Check sheet for the modelled part. Datum: model origin and axes. Units: mm. Face numbers are marked on the shaded views. A direction names the side the tool comes from. Round coordinates to 2 decimals unless told otherwise and drop trailing zeros. Loops run counter-clockwise (first coordinate to the right, second up) from the corner with the lowest first, then second, coordinate; pieces in that order, holes last. Notation, with made-up numbers: (26, 77) -> (38, 77) arc R15 ccw to (38, 102) -> close; hole circle Ø7 at (22, 58). An arc over 180 degrees is marked (long way). Return JSON: item names as keys, results as strings.
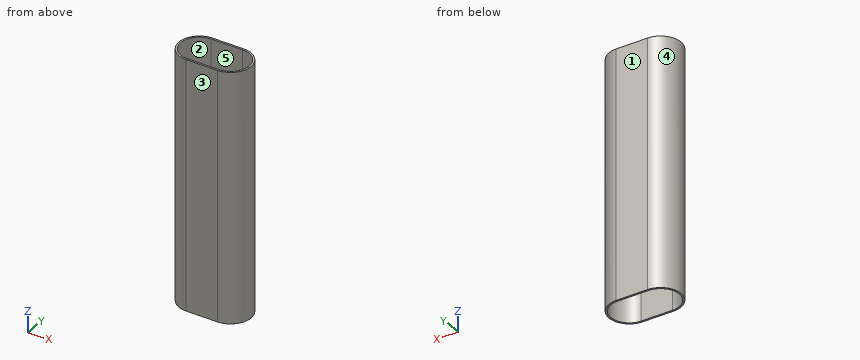
from build123d import *

# Parameters (mm, degrees)
F1_DEPTH = 85
F0_W     = 50
F0_H     = 7
F2_R     = 12.5
F2_R_2   = 7.5
F3_DEPTH = 12.5
F4_W     = 25.6223708915
F4_H     = 20
F5_DEPTH = 25


with BuildPart() as f1:
    # F0 (on Top) → F1 (new body)
    with BuildSketch(Plane.XY):
        with BuildLine():
            Line((5.35, 6.9), (-5.35, 6.9))
            ThreePointArc((-5.35, 6.9), (-12.25, 0), (-5.35, -6.9))
            Line((-5.35, -6.9), (5.35, -6.9))
            ThreePointArc((5.35, -6.9), (12.25, 0), (5.35, 6.9))
        make_face()
        with BuildLine():
            ThreePointArc((-5.35, -6.3), (-11.65, 0), (-5.35, 6.3))
            Line((-5.35, 6.3), (5.35, 6.3))
            ThreePointArc((5.35, 6.3), (11.65, 0), (5.35, -6.3))
            Line((5.35, -6.3), (-5.35, -6.3))
        make_face(mode=Mode.SUBTRACT)
    extrude(amount=F1_DEPTH)


with BuildPart() as f1b:
    # F0 (on Top) → F1, piece 2 (new body)
    with BuildSketch(Plane.XY):
        with Locations((0, -23.5)):
            Rectangle(F0_W, F0_H)
    extrude(amount=F1_DEPTH)


with BuildPart() as f3:
    # F2 (on Right) → F3 (new body, symmetric)
    with BuildSketch(Plane.YZ):
        with Locations((-35, 30)):
            Circle(F2_R)
        with Locations((-35, 30)):
            Circle(F2_R_2, mode=Mode.SUBTRACT)
    extrude(amount=F3_DEPTH, both=True)

    # F4 (on face) → F5 (join)
    with BuildSketch(Plane.YZ.offset(12.5)):
        with Locations((-42.8111854458, 34.4098300563)):
            Rectangle(F4_W, F4_H)
    extrude(amount=F5_DEPTH)


solid = f1.part
Q1. Tool access check on the marked faces 4 and 5. Record the directions out of +Z, -Z, +X, -X, +Y, -Y that give a thin tool (end or side, any length) a straight path to the whole face; none if there is none.
Results list:
{"face 4": "+Z, -Z, -X", "face 5": "+Z, -Z"}
Q2. Go/stop test with flat-tipped pins: pin 1 (2 mm diameter, centred on y = 4.5, z = 73.5, fed in from +X); pin 2 (1 mm diameter, centred on x = 8, z = 31, fed in from -Y). Record where each tip stops, or that it passes through.
Results list:
{"pin 1": "x = 11.3", "pin 2": "y = -6.56"}
Q3. Section check B-B (x = -1). Record the boundary of the cut face in (y, z), then the cut area to 3 significant figures.
Results list:
{"outline": "(-6.9, 0) -> (-6.3, 0) -> (-6.3, 85) -> (-6.9, 85) -> close; (6.3, 0) -> (6.9, 0) -> (6.9, 85) -> (6.3, 85) -> close", "area": "102 mm^2"}
Q4. Section check C-C (z = 24.5). Record the boundary of the cut face in (x, y), then the cut area to 3 significant figures.
Results list:
{"outline": "(-5.35, -6.9) -> (5.35, -6.9) arc R6.9 ccw to (5.35, 6.9) -> (-5.35, 6.9) arc R6.9 ccw to start; hole (-5.35, -6.3) -> (5.35, -6.3) arc R6.3 ccw to (5.35, 6.3) -> (-5.35, 6.3) arc R6.3 ccw to start", "area": "37.7 mm^2"}
Q5. Material ranges on line 1 (Y direction, x = 3.75, z = 11.5); line 2 (X direction, y = 0.25, z = 20); line 3 (X direction, y = -3.25, z = 38.5), recorded low to high.
Results list:
{"line 1": "-6.9 to -6.3, 6.3 to 6.9", "line 2": "-12.25 to -11.65, 11.65 to 12.25", "line 3": "-11.44 to -10.75, 10.75 to 11.44"}
Q6. Section check A-A (y = 0). Record the boundary of the cut face in (x, z), then the cut area to 3 significant figures.
Results list:
{"outline": "(-12.25, 0) -> (-11.65, 0) -> (-11.65, 85) -> (-12.25, 85) -> close; (11.65, 0) -> (12.25, 0) -> (12.25, 85) -> (11.65, 85) -> close", "area": "102 mm^2"}
Q7. Draft check along Y on the marked faces 1, 2 and 3. Enter one of: released by +Y, released by -Y, zero draft, split by the parting line, or undercut.
Results list:
{"face 1": "released by +Y", "face 2": "undercut", "face 3": "released by -Y"}
